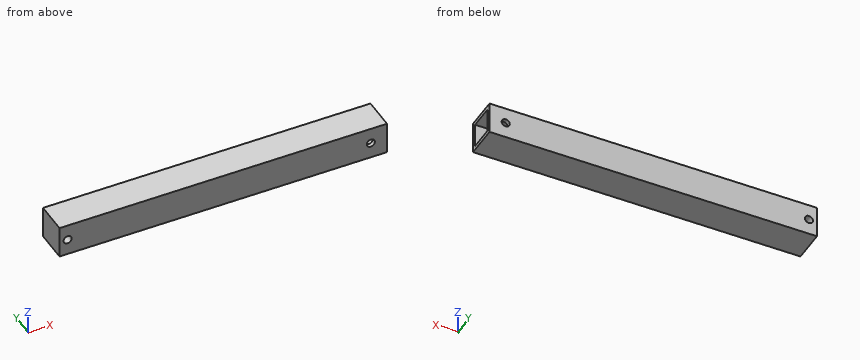
Autodesk Inventor part; units mm, degrees
ref_plane "YZ Plane" through (0, 0, 0) normal (1, 0, 0) x (0, 1, 0)
ref_plane "XZ Plane" through (0, 0, 0) normal (0, 1, 0) x (-1, 0, 0)
ref_plane "XY Plane" through (0, 0, 0) normal (0, 0, 1) x (1, 0, 0)
sketch "Sketch1" plane through (0, 0, 0) normal (0, 1, 0) x (-1, 0, 0)
  line L0 (7.8808, 9.3738) -> (-248.8624, 9.3738)
  line L1 (-248.8624, 9.3738) -> (-248.8624, -16.0262)
  line L2 (-248.8624, -16.0262) -> (7.8808, -16.0262)
  line L3 (7.8808, -16.0262) -> (7.8808, 9.3738)
  point P0 (0, 0)
  dimension "d0" = 25.4
  dimension "d1" = 256.7432
extrude "Extrusion1" add sketch "Sketch1" along normal blind 25.4
sketch "Sketch2" plane through (0, 25.4, 0) normal (0, 1, 0) x (1, 0, 0)
  line L0 (-7.8808, -9.3738) -> (248.8624, -9.3738)
  line L1 (248.8624, -9.3738) -> (248.8624, 16.0262)
  line L2 (248.8624, 16.0262) -> (-7.8808, 16.0262)
  line L3 (-7.8808, 16.0262) -> (-7.8808, -9.3738)
  circle A0 centre (-1.5308, 3.3262) radius 3.175
  circle A1 centre (236.1624, 3.3262) radius 3.175
  point P0 (0, 0)
  dimension "d4" = 6.35
  dimension "d5" = 6.35
  dimension "d6" = 237.6932
  dimension "d7" = 6.35
extrude "Extrusion2" cut sketch "Sketch2" against normal blind 25.4 contours A0 | A1
sketch "Sketch3" plane through (248.8624, 0, 9.3738) normal (1, 0, 0) x (0, 0, -1)
  line L0 (3.175, 22.225) -> (22.225, 22.225)
  line L1 (22.225, 22.225) -> (22.225, 3.175)
  line L2 (22.225, 3.175) -> (3.175, 3.175)
  line L3 (3.175, 3.175) -> (3.175, 22.225)
  line L4 (25.4, 0) -> (25.4, 25.4)
  line L5 (0, 25.4) -> (25.4, 25.4)
  line L6 (0, 0) -> (0, 25.4)
  line L7 (0, 0) -> (25.4, 0)
  point P0 (9.3738, 0)
  dimension "d10" = 3.175
  dimension "d11" = 3.175
  dimension "d12" = 3.175
  dimension "d13" = 3.175
extrude "Extrusion3" cut sketch "Sketch3" against normal blind 228.6 contours L0 L1 L2 L3
properties part number "Yarm"
Source: CAD feature listing. Evaluate the final solid. Frame: model axes, mm. Give positions to 0.01 mm unless a question says otherwise; leave off trailing zeros. Write each loop counter-clockwise with the first axis right and the second up, starting at its lowest first coordinate (ties: lowest second). Pieces come first, ordered by that corner, then holes. Notation, with made-up numbers: (54.5, 18.25) - (99.5, 18.25) arc R19 ccw to (99.5, 47.25) - close; hole circle Ø7 at (78.25, 64.5). An arc over 180 degrees is marked (long way). One line per item, written item: value. Start each with the question number.
Q1. Section query C-C, the plane y = 7.5. Return the cut outline in (x, z) (3 decimals).
Q2. First-contact query: pin 1 Ø1.5 at (y, z) = (16.5, 1) entering from +X; pin 2 Ø4 at (x, z) = (236.16, -3.33) entering from +Y. Flat tips, straight axial feed; report the tip coordinate or a pass-through.
Q3. Section query B-B, the plane x = 38. Return the cut outline in (y, z) (3 decimals), then the cut area to 3 significant figures.
Q4. Material intervals for probe 1 along Y at (x, z) = (28, -10.5) (3 decimals); probe 2 along Z at (x, y) = (97, 18.75); probe 3 along X at (y, z) = (15.75, 5.5), sorted ascending. Write a range as from..to.
Q5. Section query A-A, the plane z = -10.25. Return the cut outline in (x, y) (3 decimals).
Answer:
1. outline: (-7.881, -16.026) - (248.862, -16.026) - (248.862, -12.851) - (20.262, -12.851) - (20.262, 6.199) - (248.862, 6.199) - (248.862, 9.374) - (-7.881, 9.374) - close; hole circle Ø6.35 at (-1.531, -3.326)
2. pin 1: stops at x = 20.26
2. pin 2: passes through
3. outline: (0, -16.026) - (25.4, -16.026) - (25.4, 9.374) - (0, 9.374) - close; hole (3.175, -12.851) - (22.225, -12.851) - (22.225, 6.199) - (3.175, 6.199) - close
3. area: 282 mm2
4. probe 1: y = 0..3.175, 22.225..25.4
4. probe 2: z = -16.03..-12.85, 6.2..9.37
4. probe 3: x = -7.88..20.26
5. outline: (-7.881, 0) - (248.862, 0) - (248.862, 3.175) - (20.262, 3.175) - (20.262, 22.225) - (248.862, 22.225) - (248.862, 25.4) - (-7.881, 25.4) - close
